The model under review builds one solid part; all positions refer to its coordinate system, in mm. A direction names the side the tool comes from. Coordinates: 2 decimals unless noted, no trailing zeros. Loops run counter-clockwise (first coordinate to the right, second up) from the corner with the lowest first, then second, coordinate; pieces in that order, holes last. Notation, with made-up numbers: (15.25, -17) - (50.25, -17) arc R20 ccw to (50.25, 5) - close; hole circle Ø4 at (25, 33). An arc over 180 degrees is marked (long way). Answer in a Markdown table with one row per item. Add a question column.
(1) Machinability: for faces 4 (the cylindrical face through (-14.985, 0.66, 43.031)), 5 (the flat face through (0, 2, -4)), 6 (the flat face through (-2.5, -5, -6)), which of the approach directions +Z, -Z, +X, -X, +Y, -Y give a long, thin tool a straight path to every point of the face, cutting with its end or side? Answer none if there is none.
(2) For P1, Ø8, axis at y = -5, z = -6.5, coming from the -X side; P2, Ø5, axis at x = 14, z = 25, coming from the +Y side; P3, Ø10, axis at x = 0, y = -20.5, coming from the +Z side, all flat-tipped, find the tip position at first contact; note any pin that passes through.
(3) Mouldability with a two-part tool opening along Y and no side actions: class faces 1 (the cylindrical face through (-2.93, -13.18, 42.27)), 2 (the cylindrical face through (-0.035, 12.797, -8.859)), 3 (the flat face through (0, -16, -3)) as +Y half, -Y half, draft (parallel to the pull), parting line (faces both ways), or undercut.
(4) We need section D-D on y = -38. Write out the cut boundary in (x, z), plus the area to 3 significant figures.
(5) For line 1 along Y through (x, z) = (0, 47); line 2 along Y through (x, z) = (8, 36.5); line 3 along X through (y, z) = (5, 60.5), list the stretches that pass through material, from the lowest coordinate up.
(6) We need section A-A on y = 0. Write out the cut boundary in (x, z).
(7) We need section C-C on z = 29. Write out the cut boundary in (x, y).
from build123d import *

# Parameters (mm, degrees)
F0_W         = 50
F0_H         = 100
F1_DEPTH     = 10
F2_R         = 15
F3_DEPTH     = 67
F4_T         = -1.5
F5_R         = 12.5
F6_DEPTH     = 147
F7_SIZE      = 4
F9_DEPTH     = 10
F10_W        = 5
F10_H        = 6
F11_DEPTH    = 20
F12_R        = 4
F13_R        = 4
F14_T1_DEPTH = 22.3205080757


# Not quite as in the source:
# - a fillet or chamfer that OpenCascade refuses, or shapes differently, is made with other operations: its cross-section is extruded or revolved along the edge and cut away or added


with BuildPart() as f1:
    # F0 (on Top) → F1 (new body)
    with BuildSketch(Plane.XY):
        Rectangle(F0_W, F0_H)
    extrude(amount=F1_DEPTH)

    # F2 (on face) → F3 (join)
    with BuildSketch(Plane.XY.offset(10)):
        Circle(F2_R)
    extrude(amount=F3_DEPTH)

    # F4
    f4_openings = [f1.faces().sort_by_distance(p)[0] for p in [
        (0, 0, 77),
    ]]
    offset(amount=F4_T, openings=f4_openings, kind=Kind.INTERSECTION)

    # F5 (on face) → F6 (join)
    with BuildSketch(Plane.XY.offset(1.5)):
        Circle(F5_R)
    extrude(amount=F6_DEPTH)

    # F7
    f7_edges = [f1.edges().sort_by_distance(p)[0] for p in [
        (-12.5, 0, 148.5),
    ]]
    chamfer(f7_edges, length=F7_SIZE)

    # F8 (on face) → F9 (join)
    with BuildSketch(Plane(origin=(0, 0, 0), x_dir=(1, 0, 0), z_dir=(0, 0, -1))):
        Polygon((2.5, 16), (0, 16), (-2.5, 16), (-2.5, 6), (2.5, 6), align=None)
    extrude(amount=F9_DEPTH)

    # F10 (on face) → F11 (join)
    with BuildSketch(Plane(origin=(0, -6, 0), x_dir=(-1, 0, 0), z_dir=(0, 1, 0))):
        with Locations((0, -7)):
            Rectangle(F10_W, F10_H)
    extrude(amount=F11_DEPTH)

    # F12
    f12_edges = [f1.edges().sort_by_distance(p)[0] for p in [
        (0, 14, -10),
    ]]
    fillet(f12_edges, radius=F12_R)

    # F13
    f13_edges = [f1.edges().sort_by_distance(p)[0] for p in [
        (0, -16, -10),
    ]]
    fillet(f13_edges, radius=F13_R)

    # F14: fillet of radius 4 on 1 edges, made by hand

    # F14_s2 → F14_t1 (cut)
    with BuildSketch(Plane.YZ.offset(-11.1602540378)):
        with BuildLine():
            ThreePointArc((14, -6), (12.5358983849, -4.5358983849), (10.5358983849, -4))
            Line((10.5358983849, -4), (14, -4))
            Line((14, -4), (14, -6))
        make_face()
    extrude(amount=F14_T1_DEPTH, mode=Mode.SUBTRACT)


solid = f1.part
Outcome:
| question | item | result |
|---|---|---|
| 1 | face 4 | +Z |
| 1 | face 5 | +X, -X, +Y |
| 1 | face 6 | -Z, -X, +Y, -Y |
| 2 | P1 | x = -2.5 |
| 2 | P2 | y = 9.63 |
| 2 | P3 | z = 10 |
| 3 | face 1 | undercut |
| 3 | face 2 | +Y half |
| 3 | face 3 | -Y half |
| 4 | outline | (-25, 0) - (25, 0) - (25, 10) - (-25, 10) - close; hole (-23.5, 1.5) - (23.5, 1.5) - (23.5, 8.5) - (-23.5, 8.5) - close |
| 4 | area | 171 mm² |
| 5 | line 1 | -15 to -13.5, -12.5 to 12.5, 13.5 to 15 |
| 5 | line 2 | -12.69 to -10.87, -9.6 to 9.6, 10.87 to 12.69 |
| 5 | line 3 | -14.14 to -12.54, -11.46 to 11.46, 12.54 to 14.14 |
| 6 | outline | (-25, 0) - (25, 0) - (25, 10) - (15, 10) - (15, 77) - (13.5, 77) - (13.5, 8.5) - (23.5, 8.5) - (23.5, 1.5) - (12.5, 1.5) - (12.5, 144.5) - (8.5, 148.5) - (-8.5, 148.5) - (-12.5, 144.5) - (-12.5, 1.5) - (-23.5, 1.5) - (-23.5, 8.5) - (-13.5, 8.5) - (-13.5, 77) - (-15, 77) - (-15, 10) - (-25, 10) - close; (-2.5, -10) - (2.5, -10) - (2.5, -4) - (-2.5, -4) - close |
| 7 | outline | circle Ø30 at (0, 0); circle Ø25 at (0, 0); hole circle Ø27 at (0, 0) |
